Job drawing, mm, ordinate dimensions from the low corner. One solid piece. A direction names the side the tool comes from. Give positions to 0.01 mm unless a question says otherwise; leave off trailing zeros. Order: outer loops, then holes, each group sorted by start corner. A loop starts at its lowest first (then second) coordinate and runs counter-clockwise, first axis right, second up. Notation, with made-up numbers: M 41,73 L 73,73 A22 cw 73,101 Z; hole C 34.25,13 d7. An arc over 180 degrees is marked long. One line per question, with ' | ' between items.
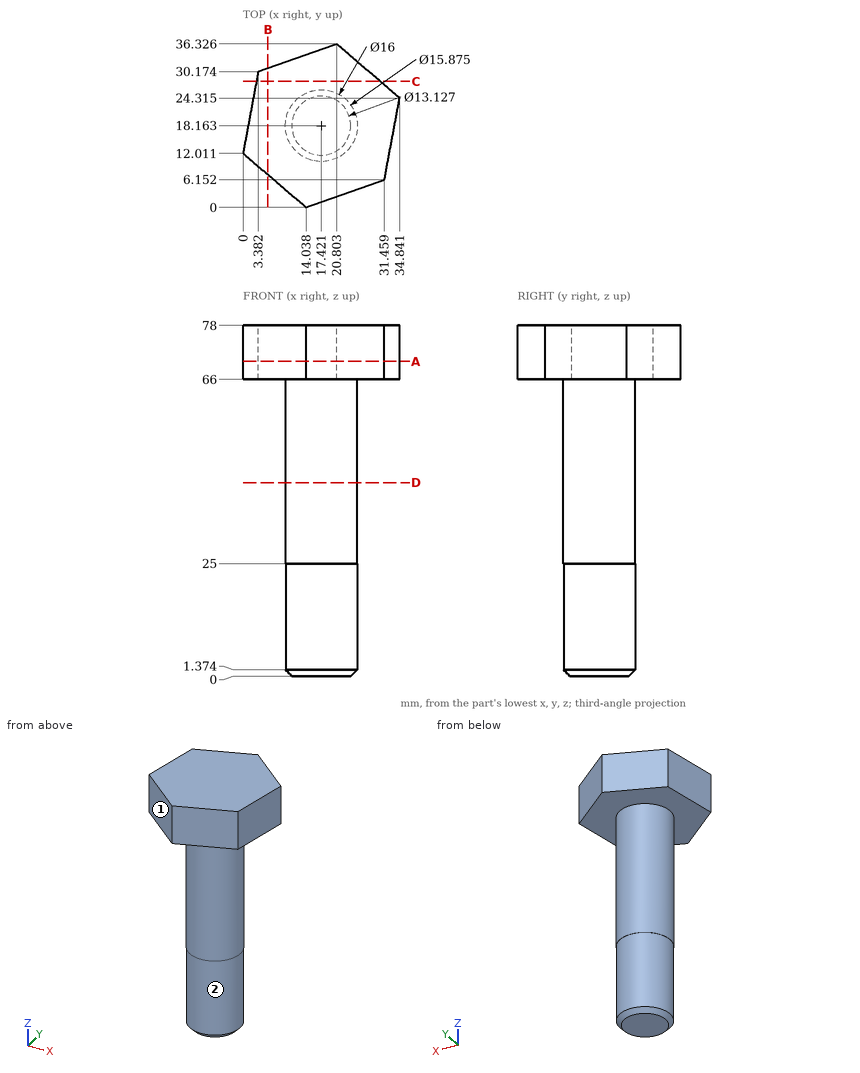
1. Tool access for the marked faces 1 and 2: list every direction of +Z, -Z, +X, -X, +Y, -Y with a clear straight run to the whole face (end or side of a thin tool).
Worked out:
face 1: +Z, -Z, -X, -Y | face 2: -Z
2. Slice it at C-C on y = 28. Give the cut face in (x, z) (1 decimal).
Worked out:
outline: M 3,66 L 30.5,66 L 30.5,78 L 3,78 Z
3. Probe L1, parallel to Z at x = 24, y = 18 (1 decimal); L2, parallel to Z at x = 13, y = 6; L3, parallel to X at y = 19, z = 34.5 (1 decimal). List the from-to ranges inside material, lowest first. Write a range as from..to.
Worked out:
L1: z = 0..78 | L2: z = 66..78 | L3: x = 9.5..25.4
4. Slice it at A-A on z = 70. Give the cut face in (x, y) (1 decimal), then the cut area to 3 significant figures.
Worked out:
outline: M 0,12 L 14,0 L 31.5,6.2 L 34.8,24.3 L 20.8,36.3 L 3.4,30.2 Z | area: 887 mm2
5. Slice it at D-D on z = 43. Give the cut face in (x, y).
Worked out:
outline: C 17.42,18.16 d16
6. Drop flat-ended pins along their axis: pin 1 (10 mm diameter, centred on y = 17.5, z = 52, fed in from -X); pin 2 (2 mm diameter, centred on y = 16, z = 45, fed in from -X) (1 decimal); pin 3 (10 mm diameter, centred on y = 25, z = 15, fed in from +X). Give the stop position or say it passes through.
Worked out:
pin 1: stops at x = 9.42 | pin 2: stops at x = 9.5 | pin 3: stops at x = 25.14
7. Slice it at B-B on x = 5.5. Give the cut face in (y, z) (1 decimal), then the cut area to 3 significant figures.
Worked out:
outline: M 7.3,66 L 30.9,66 L 30.9,78 L 7.3,78 Z | area: 283 mm2
